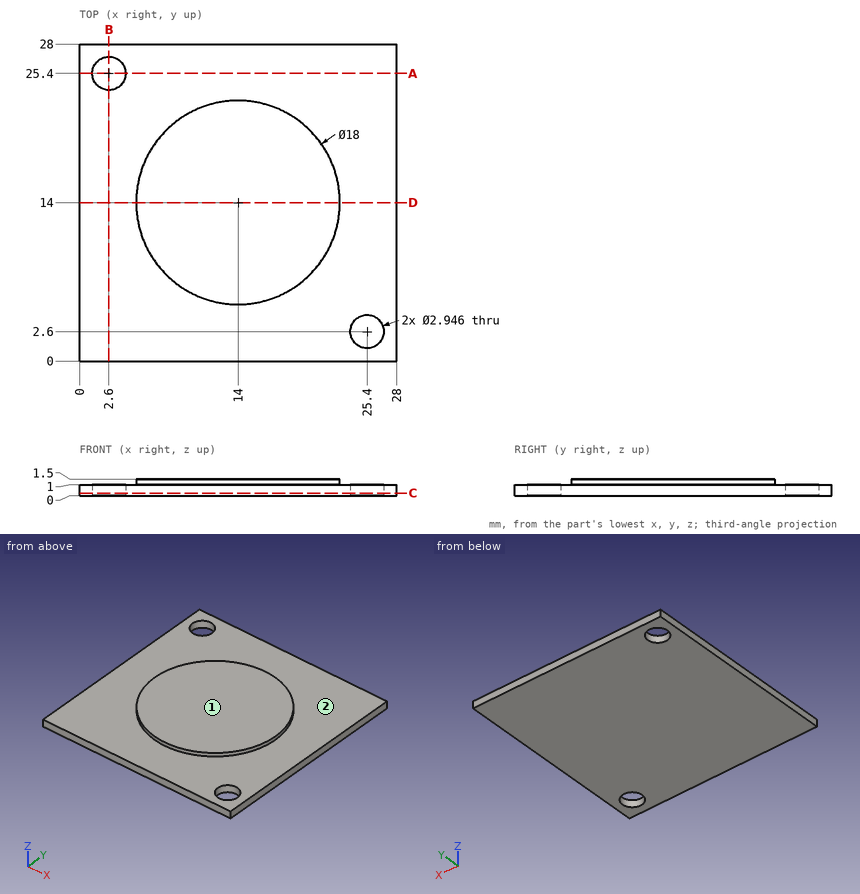
Input: dimensioned drawing with shaded views. Units: mm. Origin: part minimum x, y, z. A direction names the side the tool comes from. Coordinates: 2 decimals unless noted, no trailing zeros. Order: outer loops, then holes, each group sorted by start corner. A loop starts at its lowest first (then second) coordinate and runs counter-clockwise, first axis right, second up.
(1) Section query C-C (z = 0.25). Return the cut outline in (x, y), plus the area to 3 significant figures.
(2) Access query for the marked faces 1 and 2. Directions: +Z, -Z, +X, -X, +Y, -Y. A direction counts if a zero-diameter tool reaches every point of the face in a straight line with its end or side. Return the directions, or none.
(3) Section query B-B (x = 2.6). Return the cut outline in (y, z).
(4) Material intervals for probe 1 along Y at (x, z) = (25.4, 0.45); probe 2 along X at (y, z) = (2.5, 0.65); probe 3 along Z at (x, y) = (21.5, 2.5), sorted ascending.
(5) First-contact query: pin 1 (2.5 mm diameter, centred on x = 25.4, y = 2.6, fed in from +Z). Flat tip, straight axial feed; report the tip coordinate or a pass-through.
(6) Section query A-A (y = 25.4). Return the cut outline in (x, z).
(7) Section query D-D (y = 14). Return the cut outline in (x, z).
Solution:
1. outline: (0, 0) - (28, 0) - (28, 28) - (0, 28) - close; hole circle Ø2.95 at (2.6, 25.4); hole circle Ø2.95 at (25.4, 2.6)
1. area: 770 mm2
2. face 1: +Z, +X, -X, +Y, -Y
2. face 2: +Z
3. outline: (0, 0) - (23.93, 0) - (23.93, 1) - (0, 1) - close; (26.87, 0) - (28, 0) - (28, 1) - (26.87, 1) - close
4. probe 1: y = 0 to 1.13, 4.07 to 28
4. probe 2: x = 0 to 23.93, 26.87 to 28
4. probe 3: z = 0 to 1
5. pin 1: passes through
6. outline: (0, 0) - (1.13, 0) - (1.13, 1) - (0, 1) - close; (4.07, 0) - (28, 0) - (28, 1) - (4.07, 1) - close
7. outline: (0, 0) - (28, 0) - (28, 1) - (23, 1) - (23, 1.5) - (5, 1.5) - (5, 1) - (0, 1) - close
